Drawing for the job (mm, zero at the part's lowest x, y, z). A direction names the side the tool comes from. Give positions to 0.01 mm unless a question says otherwise; leave off trailing zeros. Write each loop counter-clockwise with the first axis right and the second up, starting at its lowest first coordinate (ties: lowest second). Pieces come first, ordered by that corner, then holes. Notation, with made-up numbers: M -37.5,49.5 L -31.5,49.5 A22 ccw -31.5,88.5 Z; hole C 21,16 d5. An arc over 180 degrees is marked long. Write item = value, one per line. Start each with the question number.
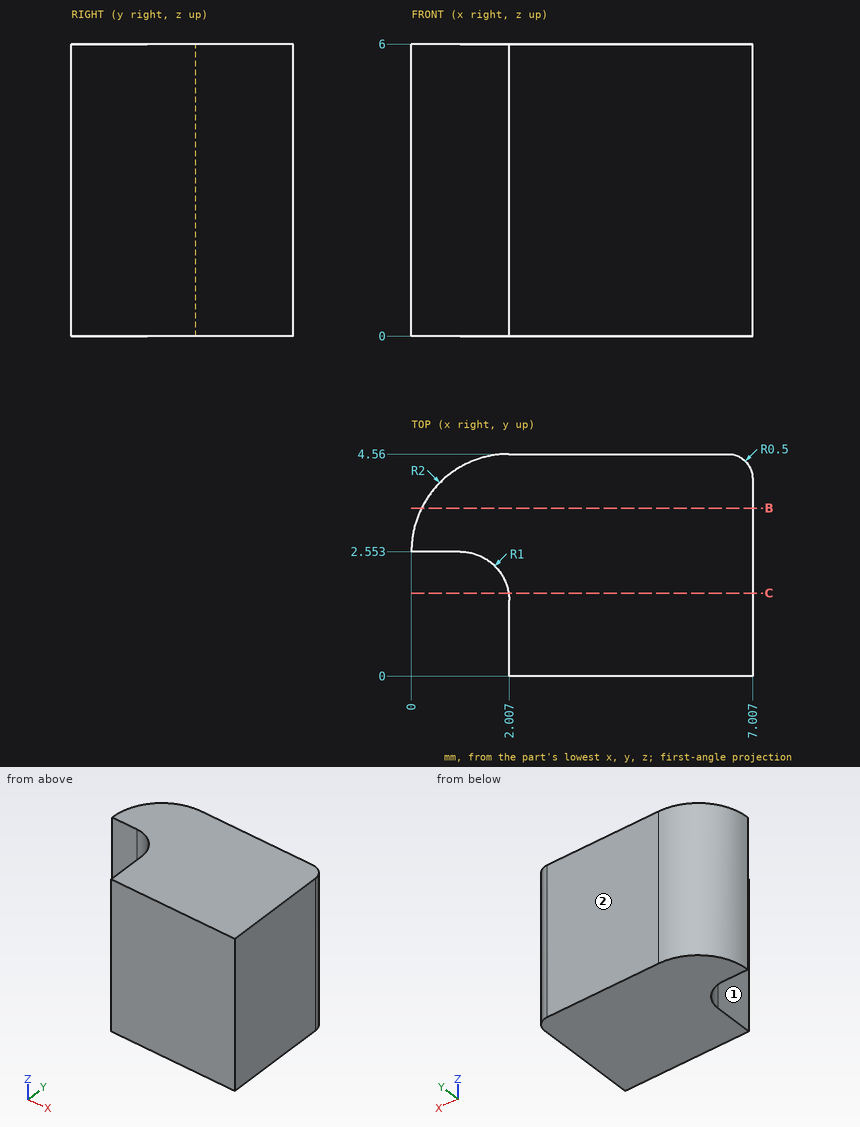
Q1. Slice it at B-B (y = 3.45). Give the cut face in (x, z), and give its area (3 significant figures).
Q2. Slice it at C-C (y = 1.7). Give the cut face in (x, z).
Q3. Drop flat-ended pins along their axis: P1, Ø1.7, axis at y = 1, z = 4, coming from the -X side; P2, Ø1.5, axis at x = 4, y = 2, coming from the -Z side. Give the stop position or say it passes through.
Q4. Tool access for the marked faces 1 and 2: list every direction of +Z, -Z, +X, -X, +Y, -Y with a clear straight run to the whole face (end or side of a thin tool).
Q5. Probe line 1 along X through (y, z) = (0.5, 3.15); line 2 along Y through (x, z) = (1.5, 5.05); line 3 along X through (y, z) = (4.25, 3.8). List the from-to ranges inside material, lowest first.
Working result:
q1.outline = M 0.21,0 L 7.01,0 L 7.01,6 L 0.21,6 Z
q1.area = 40.8 mm2
q2.outline = M 2,0 L 7.01,0 L 7.01,6 L 2,6 Z
q3.P1 = 1.96
q3.P2 = 0
q4.face_1 = +Z, -Z, -X, -Y
q4.face_2 = +Z, -Z, +X, -X, +Y
q5.line_1 = 2.01 to 7.01
q5.line_2 = 2.42 to 4.5
q5.line_3 = 0.93 to 6.97
